```python
from build123d import *

# Parameters (mm, degrees)
BASE_DEPTH                 = 88
SZKIC3_R                   = 2.5
HOLES_DEPTH                = 106.252783529
WYTNIJ_WYCI_GNI_CIE1_REACH = 107.253
SZKIC6_W                   = 3
SZKIC6_H                   = 2
WYTNIJ_WYCI_GNI_CIE3_REACH = 112.877
SZKIC7_R                   = 2.5
WYTNIJ_WYCI_GNI_CIE4_REACH = 112.877
SZKIC8_W                   = 3
SZKIC8_H                   = 2
ZAOKR_GLENIE1_R            = 1


with BuildPart() as part:
    # Szkic1 → base (new body)
    with BuildSketch(Plane.XY):
        with BuildLine():
            Line((-29.125, 0), (29.125, 0))
            ThreePointArc((29.125, 0), (37.785254038, 5), (37.785254038, 15))
            Line((37.785254038, 15), (21.350254038, 43.466255022))
            Line((21.350254038, 43.466255022), (20.484228634, 42.966255022))
            Line((20.484228634, 42.966255022), (36.919228634, 14.5))
            ThreePointArc((36.919228634, 14.5), (36.919228634, 5.5), (29.125, 1))
            Line((29.125, 1), (-29.125, 1))
            Line((-29.125, 1), (-29.125, 0))
        make_face()
    extrude(amount=BASE_DEPTH)

    # Szkic3 → holes (cut, through all)
    with BuildSketch(Plane(origin=(0, 1, 0), x_dir=(1, 0, 0), z_dir=(0, 1, 0))):
        with Locations(Location((-23.125, -3, 0), (0, 0, 270))):
            Circle(SZKIC3_R)
        with Locations(Location((-23.125, -85, 0), (0, 0, 90))):
            Circle(SZKIC3_R)
    extrude(amount=-HOLES_DEPTH, mode=Mode.SUBTRACT)

    # Szkic6 → Wytnij-wyciągnięcie1 (cut, up to next)
    with BuildSketch(Plane(origin=(0, 1, 0), x_dir=(1, 0, 0), z_dir=(0, 1, 0)), mode=Mode.PRIVATE) as wytnij_wyci_gni_cie1_sk1:
        with Locations((23.375, -84)):
            Rectangle(SZKIC6_W, SZKIC6_H)
    wytnij_wyci_gni_cie1_tool1 = extrude(wytnij_wyci_gni_cie1_sk1.sketch, amount=-WYTNIJ_WYCI_GNI_CIE1_REACH, mode=Mode.PRIVATE) & part.part
    # Szkic6 → Wytnij-wyciągnięcie1 (cut, up to next)
    with BuildSketch(Plane(origin=(0, 1, 0), x_dir=(1, 0, 0), z_dir=(0, 1, 0)), mode=Mode.PRIVATE) as wytnij_wyci_gni_cie1_sk2:
        with Locations((23.375, -4)):
            Rectangle(SZKIC6_W, SZKIC6_H)
    wytnij_wyci_gni_cie1_tool2 = extrude(wytnij_wyci_gni_cie1_sk2.sketch, amount=-WYTNIJ_WYCI_GNI_CIE1_REACH, mode=Mode.PRIVATE) & part.part
    add(wytnij_wyci_gni_cie1_tool1.solids().sort_by_distance((23.375, 1, 84))[0], mode=Mode.SUBTRACT)
    add(wytnij_wyci_gni_cie1_tool2.solids().sort_by_distance((23.375, 1, 4))[0], mode=Mode.SUBTRACT)

    # Szkic7 → Wytnij-wyciągnięcie3 (cut, up to next)
    with BuildSketch(Plane(origin=(33.968105653, 19.611494943, 0), x_dir=(0, 0, 1), z_dir=(-0.8660254037844387, -0.5000000000000001, 0)), mode=Mode.PRIVATE) as wytnij_wyci_gni_cie3_sk1:
        with Locations(Location((85, 22.464423789, 0), (0, 0, 270))):
            Circle(SZKIC7_R)
    wytnij_wyci_gni_cie3_tool1 = extrude(wytnij_wyci_gni_cie3_sk1.sketch, amount=-WYTNIJ_WYCI_GNI_CIE3_REACH, mode=Mode.PRIVATE) & part.part
    # Szkic7 → Wytnij-wyciągnięcie3 (cut, up to next)
    with BuildSketch(Plane(origin=(33.968105653, 19.611494943, 0), x_dir=(0, 0, 1), z_dir=(-0.8660254037844387, -0.5000000000000001, 0)), mode=Mode.PRIVATE) as wytnij_wyci_gni_cie3_sk2:
        with Locations(Location((3, 22.464423789, 0), (0, 0, 270))):
            Circle(SZKIC7_R)
    wytnij_wyci_gni_cie3_tool2 = extrude(wytnij_wyci_gni_cie3_sk2.sketch, amount=-WYTNIJ_WYCI_GNI_CIE3_REACH, mode=Mode.PRIVATE) & part.part
    add(wytnij_wyci_gni_cie3_tool1.solids().sort_by_distance((22.735894, 39.066257, 85))[0], mode=Mode.SUBTRACT)
    add(wytnij_wyci_gni_cie3_tool2.solids().sort_by_distance((22.735894, 39.066257, 3))[0], mode=Mode.SUBTRACT)

    # Szkic8 → Wytnij-wyciągnięcie4 (cut, up to next)
    with BuildSketch(Plane(origin=(33.968105653, 19.611494943, 0), x_dir=(0, 0, 1), z_dir=(-0.8660254037844387, -0.5000000000000001, 0)), mode=Mode.PRIVATE) as wytnij_wyci_gni_cie4_sk1:
        with Locations((44, 22.967754038)):
            Rectangle(SZKIC8_W, SZKIC8_H)
    wytnij_wyci_gni_cie4_tool1 = extrude(wytnij_wyci_gni_cie4_sk1.sketch, amount=-WYTNIJ_WYCI_GNI_CIE4_REACH, mode=Mode.PRIVATE) & part.part
    add(wytnij_wyci_gni_cie4_tool1.solids().sort_by_distance((22.484229, 39.502153, 44))[0], mode=Mode.SUBTRACT)

    # Zaokrąglenie1
    zaokr_glenie1_edges = [part.edges().sort_by_distance(p)[0] for p in [
        (22.417241336, 40.618178811, 42.5),
        (23.417241336, 38.886128003, 42.5),
        (22.417241336, 40.618178811, 45.5),
        (23.417241336, 38.886128003, 45.5),
        (21.875, 0.5, 85),
        (24.875, 0.5, 83),
        (24.875, 0.5, 85),
        (21.875, 0.5, 83),
        (21.875, 0.5, 3),
        (21.875, 0.5, 5),
        (24.875, 0.5, 3),
        (24.875, 0.5, 5),
    ]]
    fillet(zaokr_glenie1_edges, radius=ZAOKR_GLENIE1_R - 0.0001)  # a hair under: the kernel refuses the full size


solid = part.part
```
Geometry: final body of the model. Coordinates: model frame, mm. A direction names the side the tool comes from. Round coordinates to 2 decimals unless told otherwise and drop trailing zeros. Order: outer loops, then holes, each group sorted by start corner. A loop starts at its lowest first (then second) coordinate and runs counter-clockwise, first axis right, second up. Notation, with made-up numbers: M 78,-5 L 128,-5 A16 cw 128,9 Z; hole C 84.25,44.25 d5. An arc over 180 degrees is marked long. One line per item, written item: value.
(1) Cut plane C-C (x = 28). Return the cut outline in (y, z).
Result sheet:
outline: M 0,0 L 1,0 L 1,88 L 0,88 Z; M 29.95,0 L 31.95,0 L 31.95,88 L 29.95,88 Z
(2) Reachability of faces 3 (the flat face through (0, 0, 43)), 4 (the flat face through (28.59, 28.93, 43.38)) from +Z, -Z, +X, -X, +Y, -Y: full face, straight path, thin tool, end or side. Return the list, or none.
Result sheet:
face 3: +Z, -Z, +X, -X, -Y
face 4: +Z, -Z, -X
(3) Pin query (flat end, axial travel): P1, Ø12, axis at y = 27.5, z = 26, coming from the -X side; P2, Ø10, axis at y = 37, z = 75.5, coming from the -X side; P3, Ø12, axis at y = 12.5, z = 79, coming from the -X side. Return the tip coordinate at first contact, or that it passes through.
Result sheet:
P1: x = 25.95
P2: x = 21.04
P3: x = 34.61
(4) Cut plane B-B (x = -22). Return the cut outline in (y, z).
Result sheet:
outline: M 0,0 L 1,0 L 1,0.77 L 0,0.77 Z; M 0,5.23 L 1,5.23 L 1,82.77 L 0,82.77 Z; M 0,87.23 L 1,87.23 L 1,88 L 0,88 Z
(5) Pull-direction query (Z, two-part tool) for faces 1 (the cylindrical face through (24.36, 37.25, 3.75)), 2 (the flat face through (0, 1, 43)); classes: pulls with the +Z half, pulls with the -Z half, needs draft (parallel to the pull), parting line crosses it, or undercut.
Result sheet:
face 1: undercut
face 2: needs draft
(6) Line query: probe 1 along Y at (x, z) = (-4, 24.5); probe 2 along Y at (x, z) = (32.5, 69); probe 3 along Y at (x, z) = (33, 10). Output: solid intervals per line, ascending. Write a range as [from, to].
Result sheet:
probe 1: [0, 1]
probe 2: [0.59, 1.66], [22.15, 24.15]
probe 3: [0.78, 1.88], [21.29, 23.29]
(7) Cut plane D-D (y = 21). Return the cut outline in (x, z).
Result sheet:
outline: M 33.17,0 L 34.32,0 L 34.32,88 L 33.17,88 Z
(8) Cut plane A-A (z = 47). Return the cut outline in (x, y) (3 decimals).
Result sheet:
outline: M -29.125,0 L 29.125,0 A10 ccw 37.785,15 L 21.35,43.466 L 20.484,42.966 L 36.919,14.5 A9 cw 29.125,1 L -29.125,1 Z
